Read the model definition and answer for the solid it produces. Units are mm, in the model's axes. Coordinates: 2 decimals unless noted, no trailing zeros. Loops run counter-clockwise (first coordinate to the right, second up) from the corner with the lowest first, then second, coordinate; pieces in that order, holes last. Notation, with made-up numbers: (21.25, 88) - (50.25, 88) arc R6 cw to (50.25, 96) - close; hole circle Ø6 at (10, -11). An arc over 180 degrees is marked (long way). Use one line per item in the form item = value.
Autodesk Inventor part; units mm, degrees
ref_plane "YZ Plane" through (0, 0, 0) normal (1, 0, 0) x (0, 1, 0)
ref_plane "XZ Plane" through (0, 0, 0) normal (0, 1, 0) x (-1, 0, 0)
ref_plane "XY Plane" through (0, 0, 0) normal (0, 0, 1) x (1, 0, 0)
sketch "スケッチ1" plane through (0, 0, 0) normal (0, 1, 0) x (-1, 0, 0)
  circle A0 centre (0, 0) radius 5
  circle A1 centre (0, 0) radius 11
  line L0 (0, 0) -> (0, -11)
  line L1 (0, 0) -> (0, 11)
  circle A2 centre (0, 9.5) radius 4.5
  circle A3 centre (0, -9.5) radius 4.5
  circle A4 centre (2.3645, 112.8492) radius 126.872
  circle A5 centre (8.3362, 58.5776) radius 45.2805
  circle A6 centre (2.3645, 112.8492) radius 54.5992
  line L2 (62.25, 31) -> (44.25, 31)
  line L3 (44.25, 31) -> (44.25, 1)
  line L4 (44.25, 1) -> (62.25, 1)
  line L5 (62.25, 1) -> (62.25, 31)
  line L6 (0, 0) -> (13.75, 0)
  line L7 (13.75, 0) -> (13.75, -16.75)
  line L8 (13.75, -16.75) -> (0, -16.75)
  line L9 (0, -16.75) -> (0, 0)
  line L10 (70.25, 35.25) -> (36.25, 35.25)
  line L11 (36.25, 35.25) -> (36.25, -11.25)
  line L12 (36.25, -11.25) -> (70.25, -11.25)
  line L13 (70.25, -11.25) -> (70.25, 35.25)
  line L14 (70.25, 0) -> (36.25, 0)
  line L15 (0, 0) -> (36.25, 0)
  point P0 (62.25, 1)
  point P1 (0.7536, 13.9365)
  point P2 (0, 5)
  point P3 (0, -5)
  point P4 (-0.087, -13.9992)
  dimension "d4" = 253.744
  dimension "d5" = 90.561
  dimension "d0" = 10
  dimension "d1" = 22
  dimension "d2" = 9
  dimension "d3" = 9
  dimension "d7" = 18
  dimension "d8" = 30
  dimension "d9" = 13.75
  dimension "d10" = 16.75
  dimension "d11" = 46.5
  dimension "d12" = 4.25
  dimension "d13" = 8
  dimension "d14" = 34
  dimension "d15" = 11.25
  dimension "d16" = 70.25
extrude "押し出し1" add sketch "スケッチ1" along normal blind 3 contours L6 A1 A3 A0 | A0 A2 A1 L6 | A2 A1 L1 | L1 A1 A2 | A3 A1 L0 | L0 A1 A3 | L6 L7 A4 A3 A1 | A1 A2 A5 L11 L15 L6 | A1 A2 | L9 A3 A1 | A1 A3 L9 | L15 L11 A4 L7 | L14 A4 L11 | L11 A5 L3 L4 A4 L14 | L2 L5 L4 L3
fillet "フィレット1" radius 3 3 edges at (-62.25, 1.5, 1) (-62.25, 1.5, 31) (-44.25, 1.5, 31)
sketch "スケッチ4" plane through (0, 3, 0) normal (0, 1, 0) x (1, 0, 0)
  arc A0 (0, 5) -> (0.087, 13.9992) centre (0, 9.5) ccw
  arc A1 (-0.7536, -13.9365) -> (0, -5) centre (0, -9.5) ccw
  arc A2 (0, 5) -> (0, -5) centre (0, 0) ccw
  circle A3 centre (0, 0) radius 11
  point P0 (0, 11)
  point P1 (0, -11)
  point P2 (-7.7782, -7.7782)
  point P3 (-11, 0)
  point P4 (-7.7782, 7.7782)
  point P5 (0, 11)
  dimension "d29" = 22
  dimension "d56" = 180
hole "穴1" at (0, 3, -11) at (0, 3, 11) at (-7.7782, 3, 7.7782) at (-11, 3, 0) at (-7.7782, 3, -7.7782) direction (0, -1, 0) diameter 2.2 end through all
sketch "スケッチ5" plane through (0, 3, 0) normal (0, 1, 0) x (1, 0, 0)
  line L0 (-59.25, -4) -> (-47.25, -4)
  line L1 (-47.25, -4) -> (-47.25, -28)
  line L2 (-47.25, -28) -> (-59.25, -28)
  line L3 (-59.25, -28) -> (-59.25, -4)
  line L4 (-62.25, -2.8114) -> (-62.25, -28)
  line L5 (-59.25, -31) -> (-45.6995, -31)
  point P0 (0, 0)
  dimension "d37" = 3
  dimension "d38" = 3
  dimension "d39" = 12
  dimension "d40" = 24
hole "穴2" at (-59.25, 3, 28) at (-47.25, 3, 28) at (-47.25, 3, 4) at (-59.25, 3, 4) direction (0, -1, 0) diameter 2.7 end through all
properties part number "connectpart4" material "アルミニウム 6061"
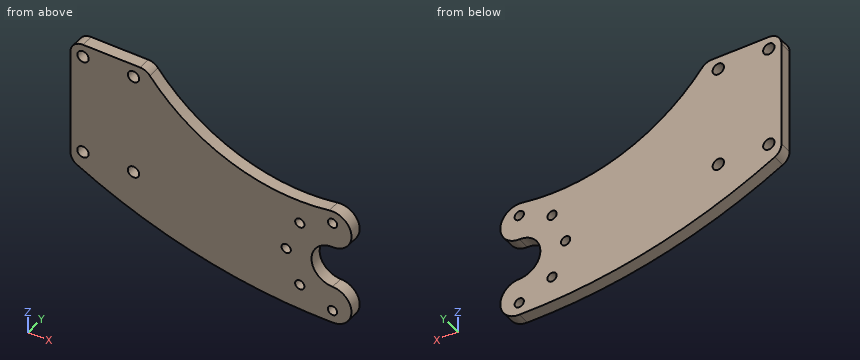
Item 1: Each of these flat-tipped pins is pushed along its axis until it touches: P1, Ø1, axis at x = -29.5, y = 2, coming from the -Z side; P2, Ø2, axis at x = 0, z = 11, coming from the -Y side; P3, Ø3.5, axis at x = 0, z = -11, coming from the -Y side. Where does it stop, or does it pass through?
Results below:
P1 = -11.2
P2 = through
P3 = 0
Item 2: Find the intervals of material crossed by L1, parallel to Z at x = -47.5, y = 0.85; L2, parallel to Z at x = -59.25, y = 1.1; L3, parallel to X at y = 0.6, z = 4, in increasing order.
Results below:
L1 = -5.72 to 2.67, 5.33 to 26.67, 29.33 to 31
L2 = -0.56 to 2.65, 5.35 to 26.65, 29.35 to 31
L3 = -62.25 to -60.6, -57.9 to -48.6, -45.9 to -3
Item 3: The part is cut by section A-A on y = 0.5. Count the separate pieces of the cut face and the enclosed holes in it, plus the area to 3 significant figures.
Results below:
separate_pieces = 1
enclosed_holes = 9
area = 1,900 mm²
Item 4: The part is cut by section B-B on z = 6. Give the vertices of the cut face in (x, y), plus the area to 3 significant figures.
Results below:
outline = (-62.25, 0) - (2.83, 0) - (2.83, 3) - (-62.25, 3) - close
area = 195 mm²
Item 5: The part is cut by section C-C on x = -51. Give the vertices of the cut face in (y, z), plus the area to 3 significant figures.
Results below:
outline = (0, -4.33) - (3, -4.33) - (3, 31) - (0, 31) - close
area = 106 mm²
